Verification items for the finished model (mm, model axes). Give positions to 0.01 mm unless a question says otherwise; leave off trailing zeros. Order: outer loops, then holes, each group sorted by start corner. A loop starts at its lowest first (then second) coordinate and runs counter-clockwise, first axis right, second up. Notation, with made-up numbers: (-32, 46.25) -> (11, 46.25) arc R29 ccw to (11, 78.25) -> close; hole circle Ø4 at (30.25, 26.5). An arc over 180 degrees is marked (long way). Return JSON: item names as keys, results as strings. Group by question number.
(1) Thickness scan on line 1 along Y through (x, z) = (-191.5, 0.65); line 2 along X through (y, z) = (-176.5, 0.6); line 3 along X through (y, z) = (-300, 1.4). Record the ranges inside material, lowest first.
(2) Depth check by flat-ended pin: pin 1 Ø5 at (x, y) = (-397, -207.46) entering from -Z. Enter the tip coordinate at first touch or a pass-through.
(3) Cross-section at B-B on x = -515. Enter the section's corners in (y, z).
(4) Cross-section at A-A on y = -169.5. Enter the section's corners in (x, z).
(5) Cross-section at D-D on z = 0.55. State how many separate pieces and enclosed holes the cut face has, then the cut area to 3 significant figures.
(6) Cross-section at C-C on y = -345.5. Enter the section's corners in (x, z), then the cut area to 3 significant figures.
from build123d import *

# Parameters (mm, degrees)
F0_W     = 717.448502
F0_H     = 378.451567
F1_DEPTH = 3.41884
F2_R     = 3.96875
F3_R     = 1.35255
F3_R_2   = 1.8288
F3_W     = 187.552764
F3_H     = 185.988784
F3_W_2   = 228.6
F3_H_2   = 93.0783
F4_DEPTH = 3.41884


with BuildPart() as f1:
    # F0 (on Top) → F1 (new body)
    with BuildSketch(Plane.XY):
        with Locations((-358.724251, -189.225783)):
            Rectangle(F0_W, F0_H)
    extrude(amount=F1_DEPTH)

    # F2
    f2_edges = [f1.edges().sort_by_distance(p)[0] for p in [
        (-717.448502, 0, 1.70942),
        (-717.448502, -378.451567, 1.70942),
        (0, -378.451567, 1.70942),
        (0, 0, 1.70942),
    ]]
    fillet(f2_edges, radius=F2_R)

    # F3 (on face) → F4 (cut, through all)
    with BuildSketch(Plane.XY.offset(3.41884)):
        with Locations((-713.479752, -3.96875)):
            Circle(F3_R)
        with Locations((-3.96875, -3.96875)):
            Circle(F3_R)
        with Locations((-713.479752, -374.482817)):
            Circle(F3_R)
        with Locations((-3.96875, -374.482817)):
            Circle(F3_R)
        with Locations((-704.147131, -309.107129)):
            Circle(F3_R)
        with Locations((-704.147131, -331.394638)):
            Circle(F3_R)
        with Locations((-422.20327, -331.394638)):
            Circle(F3_R)
        with Locations((-422.20327, -309.107129)):
            Circle(F3_R)
        with Locations((-17.15643, -374.482817)):
            Circle(F3_R_2)
        with Locations((-700.292072, -374.482817)):
            Circle(F3_R_2)
        with Locations((-700.292072, -34.632519)):
            Circle(F3_R)
        with Locations((-17.15643, -34.632519)):
            Circle(F3_R)
        with Locations((-396.99819, -49.956339)):
            Circle(F3_R_2)
        with Locations((-563.175201, -202.646375)):
            Rectangle(F3_W, F3_H)
        with Locations((-122.2375, -314.449917)):
            Rectangle(F3_W_2, F3_H_2)
        with Locations((-235.74375, -364.957817)):
            Circle(F3_R)
        with Locations((-122.2375, -364.957817)):
            Circle(F3_R)
        with Locations((-8.73125, -364.957817)):
            Circle(F3_R)
        with Locations((-235.74375, -263.942017)):
            Circle(F3_R)
        with Locations((-122.2375, -263.942017)):
            Circle(F3_R)
        with Locations((-8.73125, -263.942017)):
            Circle(F3_R)
        with Locations((-122.2375, -203.909117)):
            Rectangle(F3_W_2, F3_H_2)
        with Locations((-235.74375, -254.417017)):
            Circle(F3_R)
        with Locations((-122.2375, -254.417017)):
            Circle(F3_R)
        with Locations((-8.73125, -254.417017)):
            Circle(F3_R)
        with Locations((-8.73125, -153.401217)):
            Circle(F3_R)
        with Locations((-235.74375, -153.401217)):
            Circle(F3_R)
        with Locations((-122.2375, -153.401217)):
            Circle(F3_R)
        with Locations((-396.99819, -207.457078)):
            Circle(F3_R_2)
        with Locations((-396.99819, -364.957817)):
            Circle(F3_R_2)
    extrude(amount=-F4_DEPTH, mode=Mode.SUBTRACT)


solid = f1.part
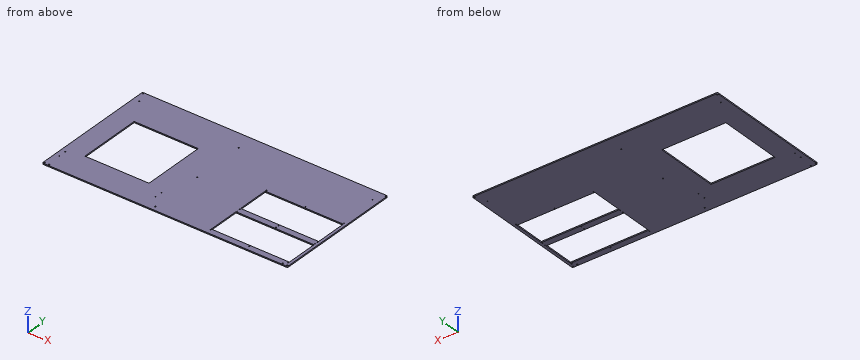
Verdict:
{
 "1": {"line 1": "-378.45 to -360.99, -267.91 to -250.45, -157.37 to 0", "line 2": "-717.45 to -656.95, -469.4 to -236.54, -7.94 to 0", "line 3": "-717.45 to -236.54, -7.94 to 0"},
 "2": {"pin 1": "z = 0"},
 "3": {"outline": "(-378.45, 0) -> (-295.64, 0) -> (-295.64, 3.42) -> (-378.45, 3.42) -> close; (-109.65, 0) -> (0, 0) -> (0, 3.42) -> (-109.65, 3.42) -> close"},
 "4": {"outline": "(-717.45, 0) -> (-656.95, 0) -> (-656.95, 3.42) -> (-717.45, 3.42) -> close; (-469.4, 0) -> (-236.54, 0) -> (-236.54, 3.42) -> (-469.4, 3.42) -> close; (-7.94, 0) -> (0, 0) -> (0, 3.42) -> (-7.94, 3.42) -> close"},
 "5": {"separate pieces": "1", "enclosed holes": "30", "area": "194,000 mm²"},
 "6": {"outline": "(-717.45, 0) -> (-236.54, 0) -> (-236.54, 3.42) -> (-717.45, 3.42) -> close; (-7.94, 0) -> (0, 0) -> (0, 3.42) -> (-7.94, 3.42) -> close", "area": "1,670 mm²"}
}
